from build123d import *

# Parameters (mm, degrees)
BOSS_EXTRUDE1_DEPTH = 12
LPATTERN1_COUNT     = 2
LPATTERN1_PITCH     = 2.5
BOSS_EXTRUDE3_DEPTH = 2.5
LPATTERN3_COUNT     = 5
LPATTERN3_PITCH     = 2.5


with BuildPart() as part:
    # Sketch1 → Boss-Extrude1 (new body)
    with BuildSketch(Plane(origin=(0, 0, 0), x_dir=(1, 0, 0), z_dir=(0, 1, 0))):
        Polygon((-0.325, 0.225), (-0.225, 0.325), (0.225, 0.325), (0.325, 0.225), (0.325, -0.225), (0.225, -0.325), (-0.225, -0.325), (-0.325, -0.225), align=None)
    extrude(amount=BOSS_EXTRUDE1_DEPTH)


with BuildPart() as lpattern1_1:
    # LPattern1: pattern copy
    add(part.part.moved(Location(Vector(1, 0, 0) * (1 * LPATTERN1_PITCH))))


with BuildPart() as part_1:
    add(part.part)

    add(lpattern1_1.part)  # Boss-Extrude3 merges LPattern1_1
    # Sketch3 → Boss-Extrude3 (add)
    with BuildSketch(Plane(origin=(0, 3, 0), x_dir=(-1, 0, 0), z_dir=(0, -1, 0))):
        Polygon((-3.75, 0.75), (-3.25, 1.25), (0.75, 1.25), (1.25, 0.75), (1.25, -0.75), (0.75, -1.25), (-3.25, -1.25), (-3.75, -0.75), align=None)
    extrude(amount=-BOSS_EXTRUDE3_DEPTH)


with BuildPart() as lpattern3_1:
    # LPattern3: pattern copy
    add(part_1.part.moved(Location(Vector(0, 0, 1) * (1 * LPATTERN3_PITCH))))


with BuildPart() as lpattern3_2:
    # LPattern3: pattern copy
    add(part_1.part.moved(Location(Vector(0, 0, 1) * (2 * LPATTERN3_PITCH))))


with BuildPart() as lpattern3_3:
    # LPattern3: pattern copy
    add(part_1.part.moved(Location(Vector(0, 0, 1) * (3 * LPATTERN3_PITCH))))


with BuildPart() as lpattern3_4:
    # LPattern3: pattern copy
    add(part_1.part.moved(Location(Vector(0, 0, 1) * (4 * LPATTERN3_PITCH))))


with BuildPart() as part_2:
    add(part_1.part)

    # Combine1: union LPattern3_1, LPattern3_2, LPattern3_3, LPattern3_4
    add(lpattern3_1.part)
    add(lpattern3_2.part)
    add(lpattern3_3.part)
    add(lpattern3_4.part)


solid = part_2.part
Part model, mm, in its own coordinate system. A direction names the side the tool comes from. Round coordinates to 2 decimals unless told otherwise and drop trailing zeros. Loops run counter-clockwise (first coordinate to the right, second up) from the corner with the lowest first, then second, coordinate; pieces in that order, holes last. Notation, with made-up numbers: (79, -30.5) - (113, -30.5) arc R20 ccw to (113, 3.5) - close; hole circle Ø9 at (4, 36.25). An arc over 180 degrees is marked (long way). Answer as a JSON object with one key per item and string values.
Item 1: Pin check, flat tips, straight feed: pin 1 (0.5 mm diameter, centred on y = 1.5, z = 5, fed in from -X) (3 decimals); pin 2 (1.5 mm diameter, centred on x = 0.5, y = 10, fed in from -Z) (3 decimals); pin 3 (3 mm diameter, centred on x = 1, z = 10, fed in from +Y). Stop position of each tip, or through.
Output:
{"pin 1": "x = -0.325", "pin 2": "z = -0.325", "pin 3": "y = 12"}
Item 2: Wall check: L1, parallel to Z at x = 2.7, y = 6 (3 decimals); L2, parallel to Z at x = -1, y = 3.75; L3, parallel to Y at x = 1.15, z = 4.25. Give the ranges that are in metal, low to high.
Output:
{"L1": "-0.325 to 0.325, 2.175 to 2.825, 4.675 to 5.325, 7.175 to 7.825, 9.675 to 10.325", "L2": "-1 to 1, 1.5 to 3.5, 4 to 6, 6.5 to 8.5, 9 to 11", "L3": "3 to 5.5"}
Item 3: Pull direction Z, two halves, no side cores. Call faces 3 (the face through (1, 4, 11.25)), 4 (the face through (3.75, 4, 0)), 5 (the face through (1, 3, 5)): pulls with the +Z half, pulls with the -Z half, needs draft (parallel to the pull), parting line crosses it, or undercut.
Output:
{"face 3": "pulls with the +Z half", "face 4": "needs draft", "face 5": "undercut"}
Item 4: Band-saw the part on A-A on y = 6. State how many separate pieces and enclosed holes the cut face has, plus the area to 4 significant figures.
Output:
{"separate pieces": "10", "enclosed holes": "0", "area": "4.025 mm2"}
Item 5: Band-saw the part on B-B on x = 0.65. List the corners of the cut face in (y, z), plus the area to 4 significant figures.
Output:
{"outline": "(3, -1.25) - (5.5, -1.25) - (5.5, 11.25) - (3, 11.25) - close", "area": "31.25 mm2"}
Item 6: Tool access for faces 1 (the face through (-1.25, 4, 2)), 2 (the face through (1, 5.5, 5)): list every direction of +Z, -Z, +X, -X, +Y, -Y with a clear straight run to the whole face (end or side of a thin tool).
Output:
{"face 1": "+Z, -Z, -X, +Y, -Y", "face 2": "+Y"}
